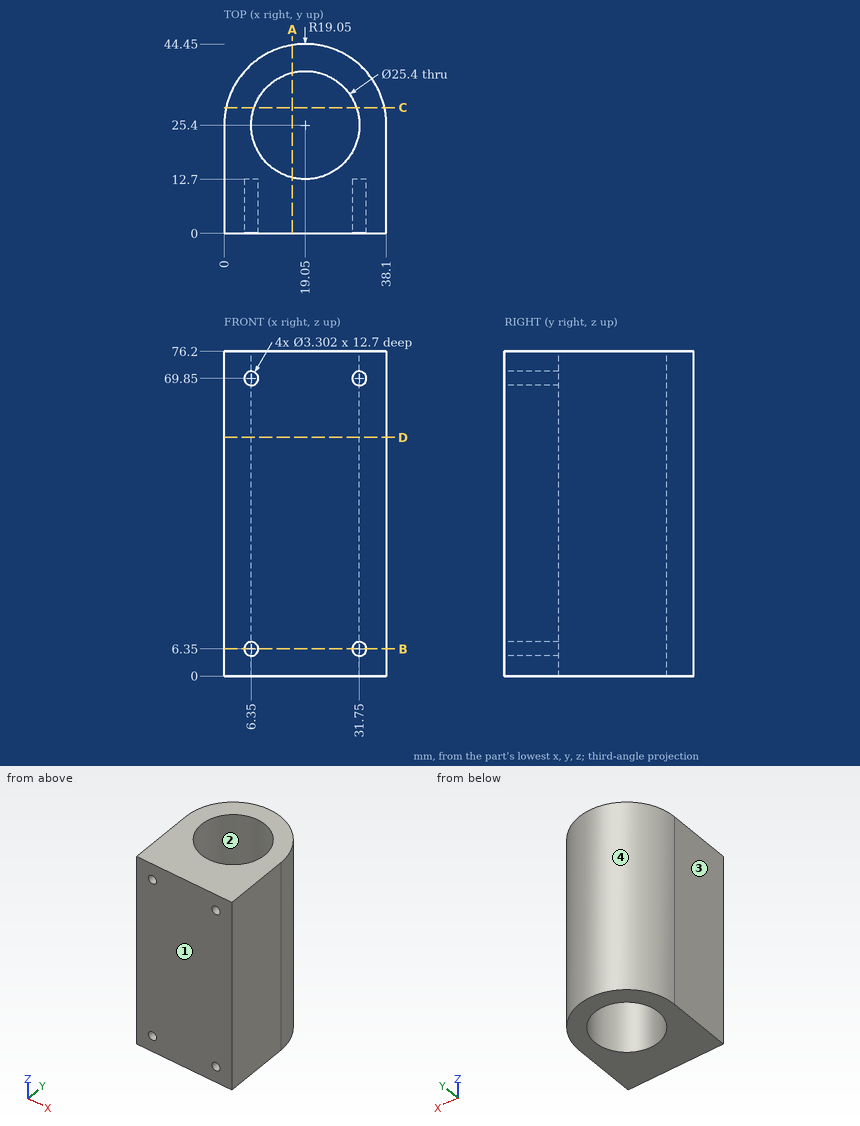
Here's the drawing with two shaded views (mm, measured from the low corner). I have some questions. Give positions to 0.01 mm unless a question says otherwise; leave off trailing zeros. Order: outer loops, then holes, each group sorted by start corner. A loop starts at its lowest first (then second) coordinate and runs counter-clockwise, first axis right, second up. Notation, with made-up numbers: (62.25, 34.5) - (112.25, 34.5) arc R20 ccw to (112.25, 57.5) - close; hole circle Ø9 at (-37.5, 73). An arc over 180 degrees is marked (long way). Use a Markdown table: item, result. Add a question column.
Q1. Please list where these lines run through material, in increasing order: line 1 along Z through (x, y) = (6.35, 10.25); line 2 along Z through (x, y) = (31, 6); line 3 along X through (y, z) = (25, 31.5).
Q2. If we mould it in two halves opening along Y, with no side actions, what happens to the marked faces 1, 2, 3 and 4? For each: released by +Y, released by -Y, zero draft, split by the parting line, or undercut.
Q3. If we section it at A-A on x = 16: Write out the boundary of the cut face in (y, z), plus the area to 3 significant figures.
Q4. I'm going to push flat-ended pins straight in: pin 1 (1 mm diameter, centred on x = 31, z = 70, fed in from -Y); pin 2 (15 mm diameter, centred on x = 19.05, y = 25.4, fed in from -Z); pin 3 (5 mm diameter, centred on y = 35, z = 62.5, fed in from -X); pin 4 (5 mm diameter, centred on x = 26.5, z = 27.5, fed in from +Y). Where does each tip first touch, or does it pass through?
Q5. If we section it at C-C on y = 29.5: Write out the boundary of the cut face in (x, z).
Q6. If we section it at B-B on z = 6.35: Write out the boundary of the cut face in (x, y), plus the area to 3 significant figures.
Q7. If we section it at D-D on z = 56: Write out the boundary of the cut face in (x, y).
Answers follow:
| question | item | result |
|---|---|---|
| 1 | line 1 | z = 0 to 4.7, 8 to 68.2, 71.5 to 76.2 |
| 1 | line 2 | z = 0 to 4.88, 7.82 to 68.38, 71.32 to 76.2 |
| 1 | line 3 | x = 0 to 6.36, 31.74 to 38.1 |
| 2 | face 1 | released by -Y |
| 2 | face 2 | undercut |
| 2 | face 3 | zero draft |
| 2 | face 4 | released by +Y |
| 3 | outline | (0, 0) - (13.07, 0) - (13.07, 76.2) - (0, 76.2) - close; (37.73, 0) - (44.2, 0) - (44.2, 76.2) - (37.73, 76.2) - close |
| 3 | area | 1,490 mm^2 |
| 4 | pin 1 | stops at y = 12.7 |
| 4 | pin 2 | passes through |
| 4 | pin 3 | stops at x = 1.37 |
| 4 | pin 4 | stops at y = 43.8 |
| 5 | outline | (0.45, 0) - (7.03, 0) - (7.03, 76.2) - (0.45, 76.2) - close; (31.07, 0) - (37.65, 0) - (37.65, 76.2) - (31.07, 76.2) - close |
| 6 | outline | (0, 0) - (4.7, 0) - (4.7, 12.7) - (8, 12.7) - (8, 0) - (30.1, 0) - (30.1, 12.7) - (33.4, 12.7) - (33.4, 0) - (38.1, 0) - (38.1, 25.4) arc R19.05 ccw to (0, 25.4) - close; hole circle Ø25.4 at (19.05, 25.4) |
| 6 | area | 947 mm^2 |
| 7 | outline | (0, 0) - (38.1, 0) - (38.1, 25.4) arc R19.05 ccw to (0, 25.4) - close; hole circle Ø25.4 at (19.05, 25.4) |
